```python
from build123d import *

# Parameters (mm, degrees)
BOSS_EXTRUDE1_DEPTH = 3
BOSS_EXTRUDE2_DEPTH = 15
SKETCH3_R           = 2
CUT_EXTRUDE1_DEPTH  = 126.116945295
SKETCH5_R           = 4
CUT_EXTRUDE3_DEPTH  = 20
CUT_EXTRUDE4_START  = -20
SKETCH6_R           = 4
CUT_EXTRUDE4_DEPTH  = 20
FILLET1_R           = 5
SKETCH7_R           = 2
CUT_EXTRUDE5_DEPTH  = 20


with BuildPart() as part:
    # Sketch1 → Boss-Extrude1 (new body)
    with BuildSketch(Plane(origin=(0, 0, 0), x_dir=(1, 0, 0), z_dir=(0, 1, 0))):
        Polygon((50, 2), (50, 11), (68, 11), (68, 21), (50, 21), (50, 37.5), (-50, 37.5), (-50, 21), (-68, 21), (-68, 11), (-50, 11), (-50, 2), (-47, 2), (-47, -2), (-50, -2), (-50, -11), (-68, -11), (-68, -21), (-50, -21), (-50, -37.5), (50, -37.5), (50, -21), (68, -21), (68, -11), (50, -11), (50, -2), (47, -2), (47, 2), align=None)
    extrude(amount=BOSS_EXTRUDE1_DEPTH)

    # Sketch2 → Boss-Extrude2 (add)
    with BuildSketch(Plane(origin=(0, 3, 0), x_dir=(1, 0, 0), z_dir=(0, 1, 0))):
        Polygon((-68, 11), (-68, 21), (-45, 21), (-45, -21), (-68, -21), (-68, -11), (-50, -11), (-50, -2), (-47, -2), (-47, 2), (-50, 2), (-50, 11), align=None)
        Polygon((45, -21), (45, 21), (68, 21), (68, 11), (50, 11), (50, 2), (47, 2), (47, -2), (50, -2), (50, -11), (68, -11), (68, -21), align=None)
    extrude(amount=BOSS_EXTRUDE2_DEPTH)

    # Sketch3 → Cut-Extrude1 (cut, through all)
    with BuildSketch(Plane.ZY.offset(50)):
        with Locations((-8.75, 13.029436278)):
            Circle(SKETCH3_R)
        with Locations((8.75, 13.029436278)):
            Circle(SKETCH3_R)
    extrude(amount=-CUT_EXTRUDE1_DEPTH, mode=Mode.SUBTRACT)

    # Sketch5 → Cut-Extrude3 (cut)
    with BuildSketch(Plane(origin=(68, 0, 0), x_dir=(0, 0, -1), z_dir=(1, 0, 0))):
        with Locations((-8.75, 13.029436278)):
            Circle(SKETCH5_R)
        with Locations((8.75, 13.029436278)):
            Circle(SKETCH5_R)
    extrude(amount=-CUT_EXTRUDE3_DEPTH, mode=Mode.SUBTRACT)

    # Sketch6 → Cut-Extrude4 (cut)
    with BuildSketch(Plane.ZY.offset(68).offset(CUT_EXTRUDE4_START)):
        with Locations(Location((8.75, 13.029436278, 0), (0, 0, 180))):
            Circle(SKETCH6_R)
        with Locations(Location((-8.75, 13.029436278, 0), (0, 0, 180))):
            Circle(SKETCH6_R)
    extrude(amount=CUT_EXTRUDE4_DEPTH, mode=Mode.SUBTRACT)

    # Fillet1
    fillet1_edges = [part.edges().sort_by_distance(p)[0] for p in [
        (47.5, 3, 21),
        (47.5, 3, -21),
        (45, 3, 0),
        (-47.5, 3, 21),
        (-45, 3, 0),
        (-47.5, 3, -21),
    ]]
    fillet(fillet1_edges, radius=FILLET1_R)

    # Sketch7 → Cut-Extrude5 (cut)
    with BuildSketch(Plane(origin=(0, 3, 0), x_dir=(1, 0, 0), z_dir=(0, 1, 0))):
        with Locations(Location((46, 33.5, 0), (0, 0, 270))):
            Circle(SKETCH7_R)
        with Locations(Location((-46, 33.5, 0), (0, 0, 270))):
            Circle(SKETCH7_R)
        with Locations(Location((46, -33.5, 0), (0, 0, 270))):
            Circle(SKETCH7_R)
        with Locations(Location((-46, -33.5, 0), (0, 0, 270))):
            Circle(SKETCH7_R)
    extrude(amount=-CUT_EXTRUDE5_DEPTH, mode=Mode.SUBTRACT)


solid = part.part
```
CAD build for the part. Positions are in the model's coordinates, mm. A direction names the side the tool comes from. Give positions to 0.01 mm unless a question says otherwise; leave off trailing zeros. Write each loop counter-clockwise with the first axis right and the second up, starting at its lowest first coordinate (ties: lowest second). Pieces come first, ordered by that corner, then holes. Notation, with made-up numbers: M -13.75,19 L 24.25,19 A23 ccw 24.25,30 Z; hole C 81,-13 d8. An arc over 180 degrees is marked long. Return JSON: item names as keys, results as strings. Group by question number.
(1) Band-saw the part on B-B (x = 58). Give the cut face in (y, z).
(2) Mould opens along Y. For faces 4 (the face through (46, 4, 23)), 5 (the face through (46.479, 11.812, -10.337)), 6 (the face through (-50, 7, -5)) say: pulls with the +Y half, pulls with the -Y half, needs draft (parallel to the pull), parting line crosses it, or undercut.
(3) Flat gauge pins, fed straight in: pin 1 Ø8 at (x, y) = (59, 4) entering from +Z; pin 2 Ø10 at (y, z) = (7, -7.5) entering from -X; pin 3 Ø6 at (x, z) = (-14, -28) entering from +Y; pin 4 Ø2 at (y, z) = (5, 0.5) entering from +X. Where does each tip first touch, or does it go through?
(4) Drill centre lines: L1, parallel to X at y = 1.3, z = 33.5; L2, parallel to X at y = 14.5, z = -16; L3, parallel to X at y = 11.75, z = -11.5. Where is each one in solid material? Low to high. Write a range as [from, to].
(5) Band-saw the part on A-A (z = 8.75). Give the cut face in (x, y).
(6) 3-axis set-ups, long thin cutter, end or side, ignore diameter. For faces 1 (the face through (55.918, 13.205, 12.746)), 2 (the face through (-50, 1, 29)), 3 (the face through (49, 9, 2)): which of +Z, -Z, +X, -X, +Y, -Y reach the whole face in a straight line?
(7) Band-saw the part on C-C (z = 18.5). Give the cut face in (x, y), and give its area (3 significant figures).
Entries:
{
 "1": {"outline": "M 0,-21 L 18,-21 L 18,-11 L 16.34,-11 A4 cw 9.72,-11 L 0,-11 Z; M 0,11 L 9.72,11 A4 cw 16.34,11 L 18,11 L 18,21 L 0,21 Z"},
 "2": {"face 4": "pulls with the +Y half", "face 5": "undercut", "face 6": "needs draft"},
 "3": {"pin 1": "stops at z = 21", "pin 2": "stops at x = -68", "pin 3": "stops at y = 3", "pin 4": "stops at x = 47"},
 "4": {"L1": "x = [-50, -48], [-44, 44], [48, 50]", "L2": "x = [-68, -45], [45, 68]", "L3": "x = [-48, -45], [45, 48]"},
 "5": {"outline": "M -50,0 L 50,0 L 50,9.03 L 48,9.03 L 48,11.03 L 45,11.03 L 45,8 A5 cw 40,3 L -40,3 A5 cw -45,8 L -45,11.03 L -48,11.03 L -48,9.03 L -50,9.03 Z; M -50,17.03 L -48,17.03 L -48,15.03 L -45,15.03 L -45,18 L -50,18 Z; M 45,15.03 L 48,15.03 L 48,17.03 L 50,17.03 L 50,18 L 45,18 Z"},
 "6": {"face 1": "+X", "face 2": "+Z, -X, +Y, -Y", "face 3": "+X, +Y, -Y"},
 "7": {"outline": "M -68,0 L 68,0 L 68,18 L 45,18 L 45,8 A5 cw 40,3 L -40,3 A5 cw -45,8 L -45,18 L -68,18 Z", "area": "1,110 mm^2"}
}
